Can you work these out from the model? Positions are in its coordinate system, mm. Coordinates: 2 decimals unless noted, no trailing zeros. Write each loop counter-clockwise with the first axis right and the second up, starting at its lowest first coordinate (ties: lowest second). Pieces come first, ordered by that corner, then holes. Notation, with made-up numbers: (77.25, 2) - (84.25, 2) arc R25 ccw to (84.25, 30) - close; hole circle Ø11 at (43.5, -15.75). An arc over 180 degrees is marked (long way). Use one line per item in the form item = value. Start each with the question number.
(1) If we section it at B-B on z = -15.5: Please give me the cut outline in (x, y), then the cut area to 3 significant figures.
(2) Thinking about a two-plate mould opening in Z: for faces 1 (the face through (38, 4, -25.8)), 2 (the face through (-18.39, 33.28, -15.94)), 3 (the face through (11.7, -35.4, -35)), which applies, pulls with the +Z half, pulls with the -Z half, needs draft (parallel to the pull), parting line crosses it, or undercut?
(3) If I drill on probe 1 along Z at (x, y) = (-28, -23); probe 2 along Y at (x, z) = (0, -26); probe 3 along Y at (x, z) = (21, -2), over which ranges is the centre line in solid material (lowest first)? Write a range as from..to.
(4) If we section it at C-C on x = 4.5: Please give me the cut outline in (y, z).
(5) For pin 1 Ø2 at (x, z) = (-16, -12.5) entering from +Y; pin 2 Ø9 at (x, y) = (-10.5, 33) entering from -Z; pin 3 Ø10 at (x, z) = (-13, -5) entering from +Y; pin 4 Ø1.5 at (y, z) = (-22, -17.5) entering from -X, each with a flat end and sliding along its axis, tell me the tip position at first contact or that it passes through.
(6) If we section it at A-A on y = -18: Please give me the cut outline in (x, z).
(7) If we section it at D-D on y = 0: Please give me the cut outline in (x, z).
```python
from build123d import *

# Parameters (mm, degrees)
F0_R     = 40
F0_R_2   = 37
F1_DEPTH = 5
F2_DEPTH = 35
F3_R     = 40
F3_R_2   = 35
F4_DEPTH = 8
F7_DEPTH = 35
F9_COUNT = 4


with BuildPart() as f1:
    # F0 (on Top) → F1 (new body)
    with BuildSketch(Plane.XY):
        Circle(F0_R)
        Circle(F0_R_2, mode=Mode.SUBTRACT)
    extrude(amount=F1_DEPTH)

    # F0 (on Top) → F2 (join)
    with BuildSketch(Plane.XY):
        Circle(F0_R)
        Circle(F0_R_2, mode=Mode.SUBTRACT)
    extrude(amount=-F2_DEPTH)

    # F3 (on Top) → F4 (join)
    with BuildSketch(Plane.XY):
        Circle(F3_R)
        Circle(F3_R_2, mode=Mode.SUBTRACT)
    extrude(amount=F4_DEPTH)

    # F9: F7 ×4 about axis
    f9_axis = Axis((0, 0, -20.4015299678), (0, 0, -1))


with BuildPart() as f7:
    # F6 (on offset) → F7 (new body)
    with BuildSketch(Plane.XZ.offset(50)):
        Polygon((3.1193340375, -5.8), (-6.2068191256, -25.8), (13.7931808744, -25.8), (23.1193340375, -5.8), align=None)
    extrude(amount=-F7_DEPTH)


with BuildPart() as f1_1:
    add(f1.part)
    for i in range(1, F9_COUNT):
        add(f7.part.rotate(f9_axis, i * 360 / F9_COUNT), mode=Mode.SUBTRACT)

    # F9#seed: cut F7
    add(f7.part, mode=Mode.SUBTRACT)


solid = f1_1.part
```
Reported:
q1.outline = (-39.98, 1.4) - (-36.97, 1.4) arc R37 cw to (-18.6, 31.99) - (-18.6, 35.41) arc R40 ccw to start; (-35.41, -18.6) arc R40 ccw to (-1.4, -39.98) - (-1.4, -36.97) arc R37 cw to (-31.99, -18.6) - close; (1.4, 36.97) arc R37 cw to (31.99, 18.6) - (35.41, 18.6) arc R40 ccw to (1.4, 39.98) - close; (18.6, -35.41) arc R40 ccw to (39.98, -1.4) - (36.97, -1.4) arc R37 cw to (18.6, -31.99) - close
q1.area = 476 mm2
q2.face_1 = undercut
q2.face_2 = undercut
q2.face_3 = pulls with the -Z half
q3.probe_1 = 0..8
q3.probe_2 = -40..-37, 37..40
q3.probe_3 = -34.04..-30.46, 30.46..34.04
q4.outline = (-39.75, -35) - (-36.73, -35) - (-36.73, -25.8) - (-39.75, -25.8) - close; (-39.75, -5.8) - (-36.73, -5.8) - (-36.73, 0) - (-34.71, 0) - (-34.71, 8) - (-39.75, 8) - close; (34.71, 0) - (36.73, 0) - (36.73, -22.14) - (39.75, -22.14) - (39.75, 8) - (34.71, 8) - close; (36.73, -35) - (39.75, -35) - (39.75, -25.8) - (36.73, -25.8) - close
q5.pin_1 = -32.86
q5.pin_2 = -35
q5.pin_3 = 39.19
q5.pin_4 = -33.89
q6.outline = (-35.72, -35) - (-32.33, -35) - (-32.33, -16.78) - (-35.72, -16.78) - close; (-35.72, -5.8) - (-32.33, -5.8) - (-32.33, 0) - (-30.02, 0) - (-30.02, 8) - (-35.72, 8) - close; (30.02, 0) - (32.33, 0) - (32.33, -35) - (35.72, -35) - (35.72, 8) - (30.02, 8) - close
q7.outline = (-40, -35) - (-37, -35) - (-37, -25.8) - (-40, -25.8) - close; (-40, -12.49) - (-37, -12.49) - (-37, 0) - (-35, 0) - (-35, 8) - (-40, 8) - close; (35, 0) - (37, 0) - (37, -12.49) - (40, -12.49) - (40, 8) - (35, 8) - close; (37, -35) - (40, -35) - (40, -25.8) - (37, -25.8) - close
